from build123d import *

# Parameters (mm, degrees)
SKETCH1_R           = 9
BASEHEAD_DEPTH      = 12
SKETCH2_R           = 6
BASEBODY_DEPTH      = 25
HEXAGONSOCKET_DEPTH = 6
TOPFILLET_R         = 1.5
CHAMFER1_SIZE       = 0.6
LPATTERN10_COUNT    = 22
LPATTERN10_PITCH    = 1.1364


with BuildPart() as part:
    # Sketch1 → BaseHead (new body)
    with BuildSketch(Plane(origin=(0, 0, 0), x_dir=(0, 0, -1), z_dir=(1, 0, 0))):
        Circle(SKETCH1_R)
    extrude(amount=BASEHEAD_DEPTH)

    # Sketch2 → BaseBody (add)
    with BuildSketch(Plane(origin=(12, 0, 0), x_dir=(0, 0, -1), z_dir=(1, 0, 0))):
        Circle(SKETCH2_R)
    extrude(amount=BASEBODY_DEPTH)

    # Sketch3 → HexagonSocket (cut)
    with BuildSketch(Plane(origin=(0, 0, 0), x_dir=(0, 0, -1), z_dir=(1, 0, 0))):
        Polygon((5.773502692, 0), (2.886751346, 5), (-2.886751346, 5), (-5.773502692, 0), (-2.886751346, -5), (2.886751346, -5), align=None)
    extrude(amount=HEXAGONSOCKET_DEPTH, mode=Mode.SUBTRACT)

    # Sketch4 → Cut-Revolve1 (revolve, cut)
    with BuildSketch(Plane(origin=(-4.19613823, 0.75, 0), x_dir=(-1, 0, 0), z_dir=(0, 0, 1))):
        Polygon((-10.19613823, 5.75), (-13.082889576, 0.75), (-10.19613823, 0.75), align=None)
    revolve(axis=Axis((0.838992387, 0, 0), (-1, 0, 0)), mode=Mode.SUBTRACT)

    # TopFillet
    topfillet_edges = [part.edges().sort_by_distance(p)[0] for p in [
        (0, 0, 9),
    ]]
    fillet(topfillet_edges, radius=TOPFILLET_R)

    # Chamfer1
    chamfer1_edges = [part.edges().sort_by_distance(p)[0] for p in [
        (37, 0, 6),
    ]]
    chamfer(chamfer1_edges, length=CHAMFER1_SIZE)

    # Sketch5 → Cut-Revolve10 (revolve, cut)
    with BuildSketch(Plane.XY):
        Polygon((36.4, 5.179873943), (36.8735, 6), (36.8735, 6.947), (35.9265, 6.947), (35.9265, 6), align=None)
    cut_revolve10 = revolve(axis=Axis((0, 0, 0), (1, 0, 0)), mode=Mode.SUBTRACT)

    # LPattern10: Cut-Revolve10 ×22
    with Locations(*[(-i * LPATTERN10_PITCH, 0, 0) for i in range(1, LPATTERN10_COUNT)]):
        add(cut_revolve10, mode=Mode.SUBTRACT)


solid = part.part
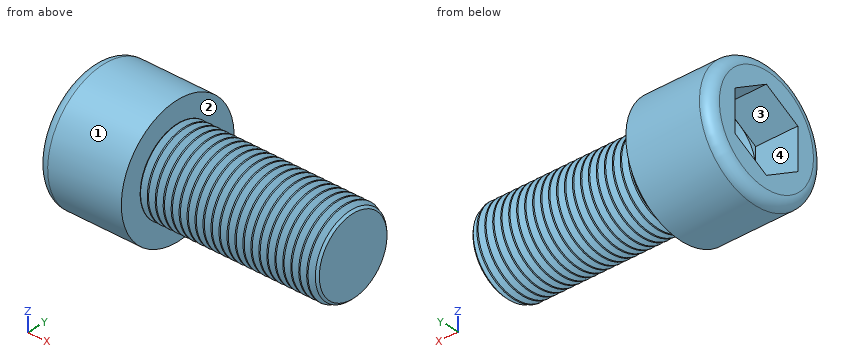
Input: part model. Units: mm. Frame: model coordinates. Face numbers are marked on the shaded views. Give positions to 0.01 mm unless a question says otherwise; leave off trailing zeros. Loops run counter-clockwise (first coordinate to the right, second up) from the corner with the lowest first, then second, coordinate; pieces in that order, holes last. Notation, with made-up numbers: M 66.25,37 L 106.25,37 A21 cw 106.25,54 Z; hole C 36,0 d5. An arc over 180 degrees is marked long. Use CSV: the item, a comma, the result in double quotes.
(1) Material intervals for L1, parallel to Z at x = 34.5, y = -3; L2, parallel to Y at x = 2.5, z = 3.25; L3, parallel to X at y = 6.75, z = 1, sorted ascending. Write a range as [from, to].
Outcome:
L1,"z = [-4.99, 4.99]"
L2,"y = [-8.39, -4.37], [4.37, 8.39]"
L3,"x = [0, 12]"
(2) Pull-direction query (Y, two-part tool) for the marked faces 1, 2, 3 and 4; classes: pulls with the +Y half, pulls with the -Y half, needs draft (parallel to the pull), parting line crosses it, or undercut.
Outcome:
face 1,"parting line crosses it"
face 2,"needs draft"
face 3,"undercut"
face 4,"undercut"
(3) Pin query (flat end, axial travel): P1, Ø3, axis at x = 6.5, y = 3.5, coming from the -Z side; P2, Ø1.5, axis at x = 14, y = -2, coming from the +Z side; P3, Ø8, axis at x = 22, z = 3, coming from the +Y side. Return the tip coordinate at first contact, or that it passes through.
Outcome:
P1,"stops at z = -8.77"
P2,"stops at z = 5.87"
P3,"stops at y = 6"
(4) Section A-A, the plane x = 5. Return loops of the section in (y, z), plus the area to 3 significant figures.
Outcome:
outline,"C 0,0 d18; hole M -5,-2.89 L 0,-5.77 L 5,-2.89 L 5,2.89 L 0,5.77 L -5,2.89 Z"
area,"168 mm²"
